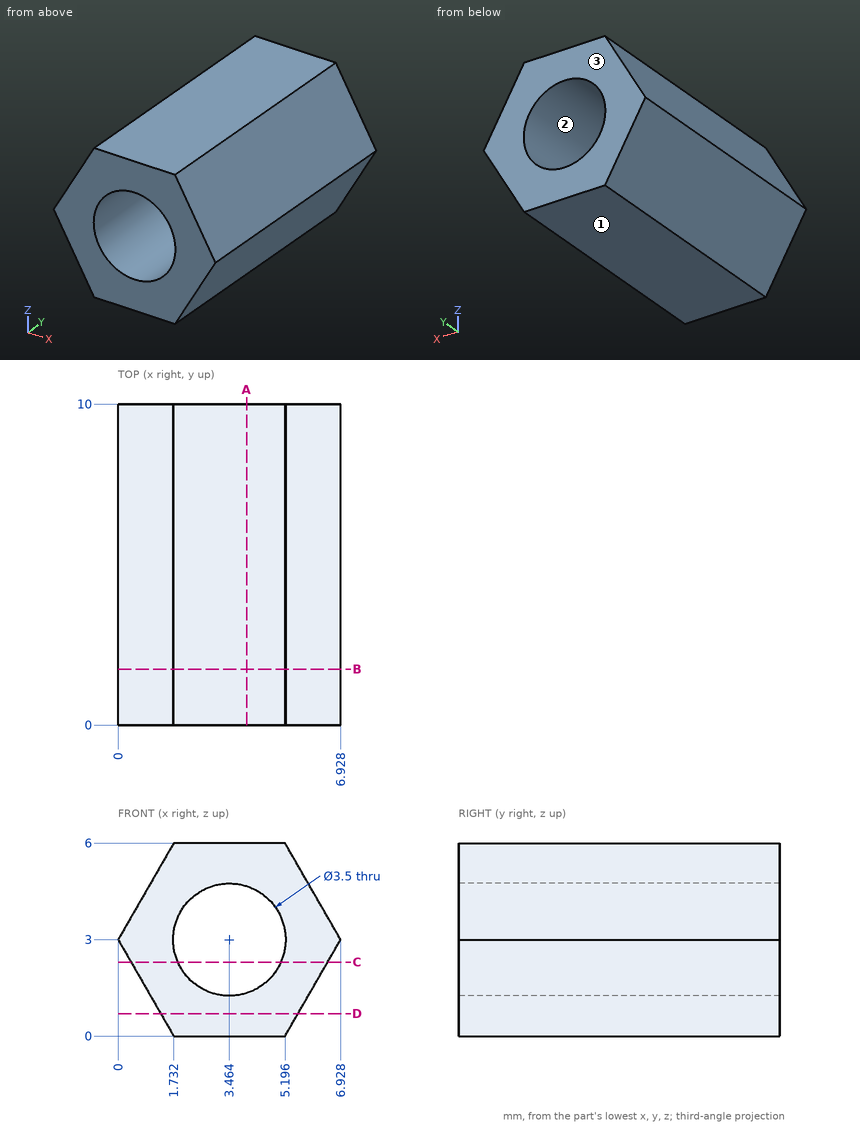
Job drawing, mm, ordinate dimensions from the low corner. One solid piece. Round coordinates to 2 decimals unless told otherwise and drop trailing zeros. Loops run counter-clockwise (first coordinate to the right, second up) from the corner with the lowest first, then second, coordinate; pieces in that order, holes last. Notation, with made-up numbers: (5, -23) -> (42, -23) arc R20 cw to (42, 9) -> close; hole circle Ø5 at (-20, 21.25). An arc over 180 degrees is marked (long way). One line per item, written item: value. Start each with the question number.
Q1. Cut at D-D on z = 0.7. List the corners of the cut face in (x, y), plus the area to 3 significant figures.
Q2. Cut at B-B on y = 1.75. List the corners of the cut face in (x, z).
Q3. Probe line 1 along Z through (x, y) = (2.5, 2.25); line 2 along Z through (x, y) = (3.5, 9.75); line 3 along X through (y, z) = (8, 4). List the from-to ranges inside material, lowest first.
Q4. Cut at A-A on x = 4. List the corners of the cut face in (y, z), plus the area to 3 significant figures.
Q5. Two-plate mould, pull along Z, no slides. Class the marked faces 1, 2 and 3: released by +Z, released by -Z, zero draft, split by the parting line, or undercut.
Q6. Cut at C-C on z = 2.3. List the corners of the cut face in (x, y), plus the area to 3 significant figures.
Q7. Drop flat-ended pins along their axis: pin 1 Ø3 at (x, z) = (3.46, 3) entering from +Y; pin 2 Ø2 at (y, z) = (8.5, 4.5) entering from -X. Give the stop position or say it passes through.
Computed:
1. outline: (1.33, 0) -> (5.6, 0) -> (5.6, 10) -> (1.33, 10) -> close
1. area: 42.7 mm²
2. outline: (0, 3) -> (1.73, 0) -> (5.2, 0) -> (6.93, 3) -> (5.2, 6) -> (1.73, 6) -> close; hole circle Ø3.5 at (3.46, 3)
3. line 1: 0 to 1.54, 4.46 to 6
3. line 2: 0 to 1.25, 4.75 to 6
3. line 3: 0.58 to 2.03, 4.9 to 6.35
4. outline: (0, 0) -> (10, 0) -> (10, 1.33) -> (0, 1.33) -> close; (0, 4.67) -> (10, 4.67) -> (10, 6) -> (0, 6) -> close
4. area: 26.7 mm²
5. face 1: released by -Z
5. face 2: undercut
5. face 3: zero draft
6. outline: (0.4, 0) -> (1.86, 0) -> (1.86, 10) -> (0.4, 10) -> close; (5.07, 0) -> (6.52, 0) -> (6.52, 10) -> (5.07, 10) -> close
6. area: 29.1 mm²
7. pin 1: through
7. pin 2: x = 0.29
